```python
from build123d import *

# Parameters (mm, degrees)
F0_W     = 10
F0_H     = 10
F0_W_2   = 8
F0_H_2   = 8
F1_DEPTH = 300
F2_W     = 10
F2_H     = 10
F3_DEPTH = 300


with BuildPart() as f1:
    # F0 (on Right) → F1 (new body)
    with BuildSketch(Plane.YZ):
        with Locations((32.823025, -4)):
            Rectangle(F0_W, F0_H)
        with Locations((32.823025, -4)):
            Rectangle(F0_W_2, F0_H_2, mode=Mode.SUBTRACT)
    extrude(amount=F1_DEPTH)

    # F2 (on face) → F3 (join)
    with BuildSketch(Plane.XY.offset(1)):
        with Locations((145, 32.823025)):
            Rectangle(F2_W, F2_H)
    extrude(amount=F3_DEPTH)


solid = f1.part
```
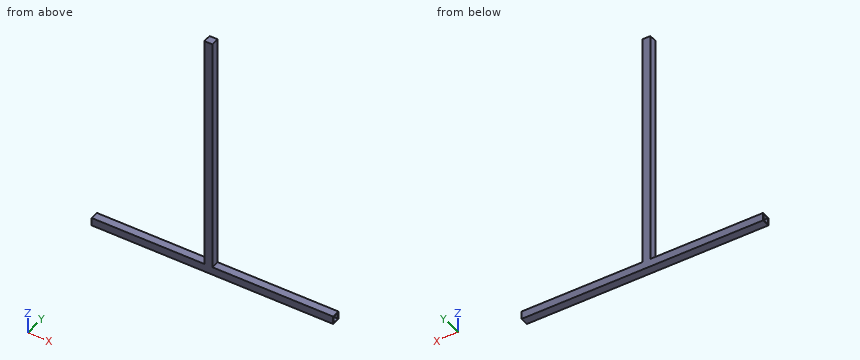
The listing builds one solid part. Answer for the finished solid, in the listing's coordinates (mm). Give positions to 0.01 mm unless a question says otherwise; leave off trailing zeros. Order: outer loops, then holes, each group sorted by start corner. A loop starts at its lowest first (then second) coordinate and runs counter-clockwise, first axis right, second up. Notation, with made-up numbers: (45.5, -9.75) -> (57.5, -9.75) arc R18 cw to (57.5, 2.25) -> close; hole circle Ø7 at (83.5, 17.5). An arc over 180 degrees is marked (long way). Write each question's results on one line, items separated by ' | '.
Q1. The part is cut by section B-B, the plane x = 29. Give the vertices of the cut face in (y, z), and give its area (3 significant figures).
Checked values:
outline: (27.82, -9) -> (37.82, -9) -> (37.82, 1) -> (27.82, 1) -> close; hole (28.82, -8) -> (36.82, -8) -> (36.82, 0) -> (28.82, 0) -> close | area: 36.0 mm^2
Q2. The part is cut by section C-C, the plane z = 90.5. Give the vertices of the cut face in (x, y).
Checked values:
outline: (140, 27.82) -> (150, 27.82) -> (150, 37.82) -> (140, 37.82) -> close
Q3. The part is cut by section A-A, the plane y = 33. Give the vertices of the cut face in (x, z), and give its area (3 significant figures).
Checked values:
outline: (0, -9) -> (300, -9) -> (300, -8) -> (0, -8) -> close; (0, 0) -> (300, 0) -> (300, 1) -> (150, 1) -> (150, 301) -> (140, 301) -> (140, 1) -> (0, 1) -> close | area: 3,600 mm^2
Q4. Each of these flat-tipped pins is pushed along its axis until it touches: P1, Ø3, axis at y = 34, z = 164, coming from the -X side; P2, Ø3, axis at x = 70.5, y = 34.5, coming from the +Z side; P3, Ø3, axis at y = 31.5, z = 114, coming from the +X side. Where does it stop, or does it pass through?
Checked values:
P1: stops at x = 140 | P2: stops at z = 1 | P3: stops at x = 150
Q5. Straight lines are drawn through the part: probe 1 along Z at (x, y) = (232.5, 35); probe 2 along Z at (x, y) = (274, 37.5); probe 3 along X at (y, z) = (31.25, 146). For each, find the intervals that lie inside material, in ascending order. Write a range as from..to.
Checked values:
probe 1: z = -9..-8, 0..1 | probe 2: z = -9..1 | probe 3: x = 140..150
